Input: dimensioned drawing with shaded views. Units: mm. Origin: part minimum x, y, z. A direction names the side the tool comes from. Round coordinates to 2 decimals unless told otherwise and drop trailing zeros. Loops run counter-clockwise (first coordinate to the right, second up) from the corner with the lowest first, then second, coordinate; pieces in that order, holes last. Notation, with made-up numbers: (54, 9.5) -> (67, 9.5) arc R22 cw to (67, 31.5) -> close; hole circle Ø11 at (72, 73.25). An arc over 180 degrees is marked (long way). Answer as a JSON object with one key per item and string values.
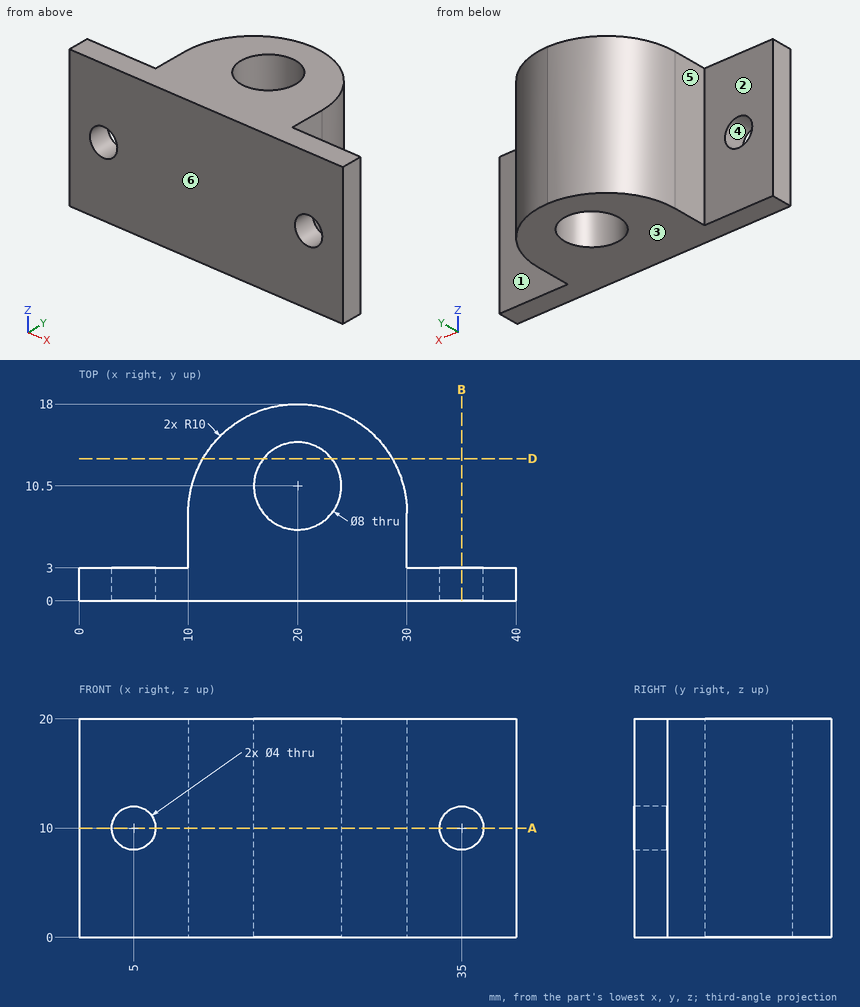
1) Section B-B, the plane x = 35. Output: boundary loops of the cut face in (y, z).
Output:
{"outline": "(0, 0) -> (3, 0) -> (3, 8) -> (0, 8) -> close; (0, 12) -> (3, 12) -> (3, 20) -> (0, 20) -> close"}
2) Draft query along X for the marked faces 4, 5 and 6. Return one class per face: +X half, -X half, draft (parallel to the pull), parting line (faces both ways), or undercut.
Output:
{"face 4": "undercut", "face 5": "-X half", "face 6": "draft"}
3) Section D-D, the plane y = 13. Output: boundary loops of the cut face in (x, z).
Output:
{"outline": "(11.34, 0) -> (16.88, 0) -> (16.88, 20) -> (11.34, 20) -> close; (23.12, 0) -> (28.66, 0) -> (28.66, 20) -> (23.12, 20) -> close"}
4) Reachability of the marked faces 1, 2 and 3 from +Z, -Z, +X, -X, +Y, -Y: full face, straight path, thin tool, end or side. Return the list, or none.
Output:
{"face 1": "+Z, -Z, +X, +Y", "face 2": "+Z, -Z, -X, +Y", "face 3": "-Z, +X, -X, +Y, -Y"}
5) Contact query for flat-ended pins moving along their axis: P1, Ø8, axis at y = 13, z = 12.5, coming from the +X side; P2, Ø5.5, axis at y = 6.5, z = 9, coming from the +X side; P3, Ø1, axis at y = 15.5, z = 14, coming from the -X side; P4, Ø5, axis at x = 21.5, y = 14, coming from the +Z side. Output: stop coordinate, or through.
Output:
{"P1": "stops at x = 29.95", "P2": "stops at x = 30", "P3": "stops at x = 12.86", "P4": "stops at z = 20"}
6) Section A-A, the plane z = 10. Count the separate pieces of the cut face and the enclosed holes in it, plus the area to 3 significant figures.
Output:
{"separate pieces": "3", "enclosed holes": "1", "area": "303 mm^2"}
7) Ray query, probe 1 along Y at (x, z) = (20, 8.25); probe 2 along Y at (x, z) = (38, 1); probe 3 along Z at (x, y) = (33.5, 1.25). Return the intervals inside material, ascending.
Output:
{"probe 1": "y = 0 to 6.5, 14.5 to 18", "probe 2": "y = 0 to 3", "probe 3": "z = 0 to 8.68, 11.32 to 20"}
